```python
from build123d import *

# Parameters (mm, degrees)
ESQUISSE2_R        = 28.5
ESQUISSE2_R_2      = 3
BOSS_EXTRU_1_DEPTH = 4


with BuildPart() as part:
    # Esquisse2 → Boss.-Extru.1 (new body)
    with BuildSketch(Plane.XY):
        with BuildLine():
            Line((40, 20), (54.641016151, 20))
            Line((54.641016151, 20), (54.641016151, -20))
            Line((54.641016151, -20), (40, -20))
            ThreePointArc((40, -20), (35.527864045, -21.05572809), (32, -24))
            ThreePointArc((32, -24), (-40, 0), (32, 24))
            ThreePointArc((32, 24), (35.527864045, 21.05572809), (40, 20))
        make_face()
        Circle(ESQUISSE2_R, mode=Mode.SUBTRACT)
        with Locations((42.141016151, 10)):
            Circle(ESQUISSE2_R_2, mode=Mode.SUBTRACT)
        with Locations(Location((42.141016151, -10, 0), (0, 0, 180))):
            Circle(ESQUISSE2_R_2, mode=Mode.SUBTRACT)
    extrude(amount=BOSS_EXTRU_1_DEPTH)


solid = part.part
```
Could you check a few things on this model? Use its own coordinates, in mm. A direction names the side the tool comes from. Coordinates: 2 decimals unless noted, no trailing zeros. Order: outer loops, then holes, each group sorted by start corner. A loop starts at its lowest first (then second) coordinate and runs counter-clockwise, first axis right, second up. Notation, with made-up numbers: M -37,-25 L 19,-25 A28 cw 19,-2 Z; hole C 66.25,-23 d3. An arc over 180 degrees is marked long. Use a Markdown table: item, result. Add a question column.
Q1. If I drill on L1, parallel to X at y = 10.5, z = 1.4; L2, parallel to Y at x = 0, z = 2.2; L3, parallel to X at y = 0.5, z = 3.65, over which ranges is the centre line in solid material (lowest first)?
Q2. I want a section at B-B on z = 3.15. List the corners of the cut face in (x, y) for me.
Q3. I want a section at A-A on x = 0. List the corners of the cut face in (y, z) for me.
Q4. I want a section at C-C on y = 0. List the corners of the cut face in (x, z) for me.
Q5. We'd pull the mould along X, two halves only. Please class faces 1 (the cylindrical face through (45.002, 10.901, 1.972)), 2 (the cylindrical face through (35.47, 21.085, 1.972)), 3 (the cylindrical face through (39.28, -10.9, 1.97)), 4 (the flat face through (47, 20, 2)): pulls with the +X half, pulls with the -X half, needs draft (parallel to the pull), parting line crosses it, or undercut.
Q6. Which directions (+Z, -Z, +X, -X, +Y, -Y) give clear straight access to the entire face, cutting with the end or side of a thin tool? Please do faces 5 (the cylindrical face through (26.327, -10.916, 1.972)), 6 (the flat face through (47, -20, 2)).
Q7. I'm going to push flat-ended pins straight in: pin 1 (5 mm diameter, centred on x = 42.14, y = 10, fed in from +Z); pin 2 (2 mm diameter, centred on x = 45.5, z = 2, fed in from -Y). Where does each tip first touch, or does it pass through?
Q8. I want a section at D-D on y = 10. List the corners of the cut face in (x, z) for me, then the cut area to 3 significant figures.
Checked values:
| question | item | result |
|---|---|---|
| 1 | L1 | -38.6 to -26.5, 26.5 to 39.18, 45.1 to 54.64 |
| 1 | L2 | -40 to -28.5, 28.5 to 40 |
| 1 | L3 | -40 to -28.5, 28.5 to 54.64 |
| 2 | outline | M 32,-24 A10 cw 40,-20 L 54.64,-20 L 54.64,20 L 40,20 A10 cw 32,24 A40 ccw long Z; hole C 0,0 d57; hole C 42.14,-10 d6; hole C 42.14,10 d6 |
| 3 | outline | M -40,0 L -28.5,0 L -28.5,4 L -40,4 Z; M 28.5,0 L 40,0 L 40,4 L 28.5,4 Z |
| 4 | outline | M -40,0 L -28.5,0 L -28.5,4 L -40,4 Z; M 28.5,0 L 54.64,0 L 54.64,4 L 28.5,4 Z |
| 5 | face 1 | undercut |
| 5 | face 2 | pulls with the +X half |
| 5 | face 3 | undercut |
| 5 | face 4 | needs draft |
| 6 | face 5 | +Z, -Z |
| 6 | face 6 | +Z, -Z, +X, -Y |
| 7 | pin 1 | through |
| 7 | pin 2 | y = -20 |
| 8 | outline | M -38.73,0 L -26.69,0 L -26.69,4 L -38.73,4 Z; M 26.69,0 L 39.14,0 L 39.14,4 L 26.69,4 Z; M 45.14,0 L 54.64,0 L 54.64,4 L 45.14,4 Z |
| 8 | area | 136 mm² |
